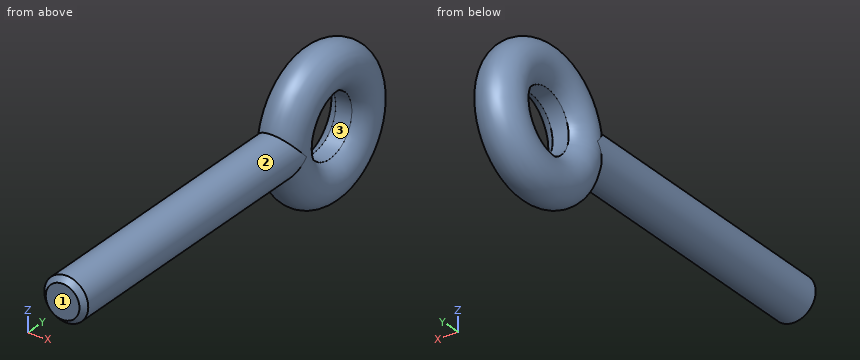
```python
from build123d import *

# Parameters (mm, degrees)
VARREDURA_DA_ARGOLA_PROFILE_R = 2.15
VARREDURA_DO_PINO_PROFILE_R   = 2.15
CHANFRO_DO_PINO_SIZE          = 0.5
ESBO_O1_R                     = 3
ESBO_O1_R_2                   = 2.85
CORTE_EXTRUS_O1_DEPTH         = 36.787497843
CORTE_EXTRUS_O1_DEPTH_BACK    = 36.787497843


with BuildPart() as part:
    # Varredura da Argola: sweep along a path in Argola
    with BuildLine(Plane(origin=(0, 0, 0), x_dir=(0, 0, -1), z_dir=(1, 0, 0))) as varredura_da_argola_path:
        CenterArc((0, 0), 5, 0, 360)
    # Varredura da Argola profile (on start of the path) → Varredura da Argola (sweep)
    with BuildSketch(Plane(origin=(0, 0, -5), x_dir=(0, 0, 1), z_dir=(0, 1, 0))):
        Circle(VARREDURA_DA_ARGOLA_PROFILE_R)
    sweep(path=varredura_da_argola_path.line)

    # Varredura do Pino: sweep along a path in Pino
    with BuildLine(Plane(origin=(0, 0, 0), x_dir=(0, 0, -1), z_dir=(1, 0, 0))) as varredura_do_pino_path:
        Line((0, -5), (0, -35))
    # Varredura do Pino profile (on start of the path) → Varredura do Pino (sweep)
    with BuildSketch(Plane(origin=(0, -5, 0), x_dir=(0, 0, -1), z_dir=(0, -1, 0))):
        Circle(VARREDURA_DO_PINO_PROFILE_R)
    sweep(path=varredura_do_pino_path.line)

    # Chanfro do pino
    chanfro_do_pino_edges = [part.edges().sort_by_distance(p)[0] for p in [
        (0, -35, 2.15),
    ]]
    chamfer(chanfro_do_pino_edges, length=CHANFRO_DO_PINO_SIZE)

    # Esbo_o1 → Corte-extrus_o1 (cut, two sides)
    with BuildSketch(Plane(origin=(0, 0, 0), x_dir=(0, 0, -1), z_dir=(1, 0, 0))) as corte_extrus_o1_sk:
        Circle(ESBO_O1_R)
        Circle(ESBO_O1_R_2, mode=Mode.SUBTRACT)
    extrude(amount=CORTE_EXTRUS_O1_DEPTH, mode=Mode.SUBTRACT)
    extrude(corte_extrus_o1_sk.sketch, amount=-CORTE_EXTRUS_O1_DEPTH_BACK, mode=Mode.SUBTRACT)


solid = part.part
```
Geometry: final body of the model. Coordinates: model frame, mm. Face numbers are marked on the shaded views. Give positions to 0.01 mm unless a question says otherwise; leave off trailing zeros. Loops run counter-clockwise (first coordinate to the right, second up) from the corner with the lowest first, then second, coordinate; pieces in that order, holes last. Notation, with made-up numbers: (60, 56.5) -> (105, 56.5) arc R5 ccw to (105, 62.5) -> close; hole circle Ø4 at (22.5, 66.25). An arc over 180 degrees is marked (long way). Use CSV: the item, a comma, the result in double quotes.
(1) Cut plane D-D (y = -31). Output: boundary loops of the cut face in (x, z), plus the area to 3 significant figures.
From the geometry:
outline,"circle Ø4.3 at (0, 0)"
area,"14.5 mm^2"
(2) Cut plane B-B (x = 0). Output: boundary loops of the cut face in (y, z).
From the geometry:
outline,"(-35, -1.65) -> (-34.5, -2.15) -> (-6.82, -2.15) arc R7.15 ccw (long way) to (-6.82, 2.15) -> (-34.5, 2.15) -> (-35, 1.65) -> close; hole circle Ø6 at (0, 0)"
(3) Cut plane C-C (y = 0). Output: boundary loops of the cut face in (x, z), plus the area to 3 significant figures.
From the geometry:
outline,"(-0.79, -3) arc R2.15 ccw (long way) to (0.79, -3) -> close; (-0.79, 3) -> (0.79, 3) arc R2.15 ccw (long way) to start"
area,"28.7 mm^2"
(4) First-contact query: P1, Ø1.5, axis at y = -25.5, z = 3.5, coming from the +X side; P2, Ø1.5, axis at y = -8.5, z = -0.5, coming from the +X side. Flat tips, straight axial feed; report the tip coordinate or a pass-through.
From the geometry:
P1,"through"
P2,"x = 2.15"
(5) Pull-direction query (Y, two-part tool) for the marked faces 1, 2 and 3; classes: released by +Y, released by -Y, zero draft, split by the parting line, or undercut.
From the geometry:
face 1,"released by -Y"
face 2,"zero draft"
face 3,"undercut"
(6) Ray query, line 1 along Y through (x, z) = (-0.1, 0); line 2 along Z through (x, y) = (0.1, 0); line 3 along Y through (x, z) = (-1.45, -2.25). Return the intervals inside material, ascending. Write a range as [from, to].
From the geometry:
line 1,"[-35, -3], [3, 7.15]"
line 2,"[-7.15, -3], [3, 7.15]"
line 3,"[-6.19, -2.57], [2.57, 6.19]"
(7) Cut plane A-A (z = 0). Output: boundary loops of the cut face in (x, y), plus the area to 3 significant figures.
From the geometry:
outline,"(-2.15, -34.5) -> (-1.65, -35) -> (1.65, -35) -> (2.15, -34.5) -> (2.15, -5) arc R2.15 ccw to (0.79, -3) -> (-0.79, -3) arc R2.15 ccw to (-2.15, -5) -> close; (-0.79, 3) -> (0.79, 3) arc R2.15 ccw (long way) to start"
area,"150 mm^2"
